Geometry: final body of the model. Coordinates: model frame, mm. A direction names the side the tool comes from. Give positions to 0.01 mm unless a question says otherwise; leave off trailing zeros. Loops run counter-clockwise (first coordinate to the right, second up) from the corner with the lowest first, then second, coordinate; pieces in that order, holes last. Notation, with made-up numbers: (50.25, 33) -> (65.25, 33) arc R9 ccw to (65.25, 47) -> close; hole circle Ø5 at (41.25, 32.25). An arc over 180 degrees is marked (long way). One line per question, with ' | ' between items. Start each with the question number.
Item 1: Section D-D on y = 6. Return loops of the section in (x, z), then the cut area to 3 significant figures.
Item 2: Section C-C on z = 12.5. Return loops of the section in (x, y).
Item 3: Section A-A on z = 0. Return loops of the section in (x, y), then the cut area to 3 significant figures.
Item 4: Mould query, pull axis X, two halves, no side actions, for faces 4 (the cylindrical face through (-22.532, 0.401, 0.82)), 5 (the cylindrical face through (-4.897, -0.751, -1.087)), 6 (the cylindrical face through (-24.638, 0.401, 0.044)). Classes: released by +X, released by -X, zero draft, split by the parting line, or undercut.
Item 5: Section B-B on x = 0. Return loops of the section in (y, z).
Item 6: Material intervals for line 1 along X through (y, z) = (0.2, 0); line 2 along Y through (x, z) = (-1.5, -3.5); line 3 along Y through (x, z) = (-18.5, 5.5), sorted ascending. Write a range as [from, to].
Item 7: Set-up query: faces 1 (the cylindrical face through (-2.55, -6.962, 3.326)), 2 (the flat face through (-17.411, 0.401, 8.033)), 3 (the flat face through (-1, -5.334, -1)). Return all of +Z, -Z, +X, -X, +Y, -Y with unobstructed straight access to the full face (end or side cutting, diameter ignored); none if empty.
Item 8: Pin query (flat end, axial travel): P1, Ø5, axis at x = -19.5, z = -12.5, coming from the +Y side; P2, Ø4.5, axis at x = 20.955, z = 0, coming from the -Y side; P3, Ø4, axis at x = -18.5, y = 1.5, coming from the +Z side; P4, Ø6.5, axis at x = -21.5, z = -1, coming from the +Y side. Return the tip coordinate at first contact, or that it passes through.
from build123d import *
from build123d.topology import SkipClean

# Parameters (mm, degrees)
SKETCH1_R           = 1.778
BOSS_EXTRUDE1_DEPTH = 0.8128
SKETCH2_R           = 17.5387
BOSS_EXTRUDE2_DEPTH = 7.8232
SKETCH3_R           = 5.0165
BOSS_EXTRUDE3_DEPTH = 1.524
SKETCH5_R           = 1.016
BOSS_EXTRUDE4_DEPTH = 3.81
SKETCH6_R           = 4.191
BOSS_EXTRUDE5_DEPTH = 3.302


with BuildPart() as part:
    # Sketch1 → Boss-Extrude1 (new body)
    with BuildSketch(Plane(origin=(0, 0, 0), x_dir=(1, 0, 0), z_dir=(0, 1, 0))):
        with BuildLine():
            Line((-23.390244242, 2.762982895), (-11.59680103, 13.157515098))
            ThreePointArc((-11.59680103, 13.157515098), (0, 17.5387), (11.59680103, 13.157515098))
            Line((11.59680103, 13.157515098), (23.390244242, 2.762982895))
            ThreePointArc((23.390244242, 2.762982895), (24.638, 0), (23.390244242, -2.762982895))
            Line((23.390244242, -2.762982895), (11.59680103, -13.157515098))
            ThreePointArc((11.59680103, -13.157515098), (0, -17.5387), (-11.59680103, -13.157515098))
            Line((-11.59680103, -13.157515098), (-23.390244242, -2.762982895))
            ThreePointArc((-23.390244242, -2.762982895), (-24.638, 0), (-23.390244242, 2.762982895))
        make_face()
        with Locations(Location((-20.955, 0, 0), (0, 0, 270))):
            Circle(SKETCH1_R, mode=Mode.SUBTRACT)
        with Locations(Location((20.955, 0, 0), (0, 0, 90))):
            Circle(SKETCH1_R, mode=Mode.SUBTRACT)
    extrude(amount=BOSS_EXTRUDE1_DEPTH)

    # Sketch2 → Boss-Extrude2 (add)
    with SkipClean():  # the faces are left unmerged after this step: merging them gives an invalid solid
        with BuildSketch(Plane(origin=(0, 0.8128, 0), x_dir=(1, 0, 0), z_dir=(0, 1, 0))):
            with Locations(Location((0, 0, 0), (0, 0, 90))):
                Circle(SKETCH2_R)
        extrude(amount=BOSS_EXTRUDE2_DEPTH)

    # Sketch3 → Boss-Extrude3 (add)
    with SkipClean():  # the faces are left unmerged after this step: merging them gives an invalid solid
        with BuildSketch(Plane(origin=(0, 0, 0), x_dir=(1, 0, 0), z_dir=(0, 1, 0))):
            with Locations(Location((0, 0, 0), (0, 0, 270))):
                Circle(SKETCH3_R)
        extrude(amount=-BOSS_EXTRUDE3_DEPTH)

    # Sketch5 → Boss-Extrude4 (add)
    with SkipClean():  # the faces are left unmerged after this step: merging them gives an invalid solid
        with BuildSketch(Plane.XZ.offset(1.524)):
            with Locations(Location((0, 0, 0), (0, 0, 90))):
                Circle(SKETCH5_R)
        extrude(amount=BOSS_EXTRUDE4_DEPTH)

    # Sketch6 → Boss-Extrude5 (add)
    with SkipClean():  # the faces are left unmerged after this step: merging them gives an invalid solid
        with BuildSketch(Plane.XZ.offset(5.334)):
            with Locations(Location((0, 0, 0), (0, 0, 270))):
                Circle(SKETCH6_R)
        extrude(amount=BOSS_EXTRUDE5_DEPTH)


solid = part.part
Result sheet:
1) outline: circle Ø35.08 at (0, 0) | area: 966 mm²
2) outline: (-12.34, 0) -> (12.34, 0) -> (12.34, 0.81) -> (12.3, 0.81) -> (12.3, 8.64) -> (-12.3, 8.64) -> (-12.3, 0.81) -> (-12.34, 0.81) -> close
3) outline: (-24.64, 0) -> (-22.73, 0) -> (-22.73, 0.81) -> (-24.64, 0.81) -> close; (-19.18, 0) -> (-5.02, 0) -> (-5.02, -1.52) -> (-1.02, -1.52) -> (-1.02, -5.33) -> (-4.19, -5.33) -> (-4.19, -8.64) -> (4.19, -8.64) -> (4.19, -5.33) -> (1.02, -5.33) -> (1.02, -1.52) -> (5.02, -1.52) -> (5.02, 0) -> (19.18, 0) -> (19.18, 0.81) -> (17.54, 0.81) -> (17.54, 8.64) -> (-17.54, 8.64) -> (-17.54, 0.81) -> (-19.18, 0.81) -> close; (22.73, 0) -> (24.64, 0) -> (24.64, 0.81) -> (22.73, 0.81) -> close | area: 359 mm²
4) face 4: undercut | face 5: split by the parting line | face 6: released by -X
5) outline: (-8.64, -4.19) -> (-5.33, -4.19) -> (-5.33, -1.02) -> (-1.52, -1.02) -> (-1.52, -5.02) -> (0, -5.02) -> (0, -17.54) -> (8.64, -17.54) -> (8.64, 17.54) -> (0, 17.54) -> (0, 5.02) -> (-1.52, 5.02) -> (-1.52, 1.02) -> (-5.33, 1.02) -> (-5.33, 4.19) -> (-8.64, 4.19) -> close
6) line 1: x = [-24.64, -22.73], [-19.18, 19.18], [22.73, 24.64] | line 2: y = [-8.64, -5.33], [-1.52, 8.64] | line 3: y = [0, 0.81]
7) face 1: -Y | face 2: +Z, -X, +Y, -Y | face 3: none
8) P1: passes through | P2: stops at y = 0 | P3: stops at z = 8.73 | P4: stops at y = 0.81
